Build history of the part. All positions in model axes, mm. Face numbers are marked on the shaded views. A direction names the side the tool comes from. Round coordinates to 2 decimals unless told otherwise and drop trailing zeros. Loops run counter-clockwise (first coordinate to the right, second up) from the corner with the lowest first, then second, coordinate; pieces in that order, holes last. Notation, with made-up numbers: M 87,12.25 L 121,12.25 A20 ccw 121,51.25 Z; hole C -24,40.5 d6. An arc over 180 degrees is marked long. Write each question's results on one line, items separated by ' | '. Start each with the question number.
```python
from build123d import *

# Parameters (mm, degrees)
SLEEVE_DEPTH       = 63.5
SLEEVE_DEPTH_BACK  = 5
SKETCH1_R          = 9.525
SKETCH2_W          = 19.05
SKETCH2_H          = 6.35
BRACKET_DEPTH      = 122
SKETCH4_R          = 5.1
BRACKET_HOLE_DEPTH = 138.86578845
SKETCH5_R          = 6.35
SHAFT_DEPTH        = 75
SKETCH6_R          = 8.73125
SLEEVE_HOLE_DEPTH  = 157.656471388
FILLET1_R          = 5


with BuildPart() as part:
    # Sketch1 → Sleeve (new, two sides: drawn at the far end of the back side and taken through both)
    with BuildSketch(Plane(origin=(0, 0, 0), x_dir=(1, 0, 0), z_dir=(0, 1, 0)).offset(-SLEEVE_DEPTH_BACK)):
        with Locations(Location((0, 0, 0), (0, 0, 270))):
            Circle(SKETCH1_R)
    extrude(amount=SLEEVE_DEPTH + SLEEVE_DEPTH_BACK)

    # Sketch2 → Bracket (add)
    with BuildSketch(Plane.XY):
        with Locations((0, 53.5)):
            Rectangle(SKETCH2_W, SKETCH2_H)
    extrude(amount=BRACKET_DEPTH)

    # Sketch4 → Bracket Hole (cut, through all)
    with BuildSketch(Plane(origin=(0, 0, 0), x_dir=(1, 0, 0), z_dir=(0, 1, 0))):
        with Locations(Location((0, -50.8, 0), (0, 0, 90))):
            Circle(SKETCH4_R)
        with Locations(Location((0, -66.1, 0), (0, 0, 90))):
            Circle(SKETCH4_R)
        with Locations(Location((0, -81.4, 0), (0, 0, 90))):
            Circle(SKETCH4_R)
        with Locations(Location((0, -96.7, 0), (0, 0, 90))):
            Circle(SKETCH4_R)
        with Locations(Location((0, -112, 0), (0, 0, 90))):
            Circle(SKETCH4_R)
    extrude(amount=BRACKET_HOLE_DEPTH, mode=Mode.SUBTRACT)

    # Sketch5 → Shaft (add)
    with BuildSketch(Plane(origin=(0, 0, 0), x_dir=(0, 0, -1), z_dir=(1, 0, 0))):
        with Locations(Location((0, 10, 0), (0, 0, 180))):
            Circle(SKETCH5_R)
    extrude(amount=SHAFT_DEPTH)

    # Sketch6 → Sleeve Hole (cut, through all)
    with BuildSketch(Plane(origin=(0, 0, 0), x_dir=(1, 0, 0), z_dir=(0, 1, 0))):
        with Locations(Location((0, 0, 0), (0, 0, 270))):
            Circle(SKETCH6_R)
    extrude(amount=SLEEVE_HOLE_DEPTH, mode=Mode.SUBTRACT)

    # Fillet1
    fillet1_edges = [part.edges().sort_by_distance(p)[0] for p in [
        (-9.525, 53.5, 122),
        (9.525, 53.5, 122),
    ]]
    fillet(fillet1_edges, radius=FILLET1_R)


solid = part.part
```
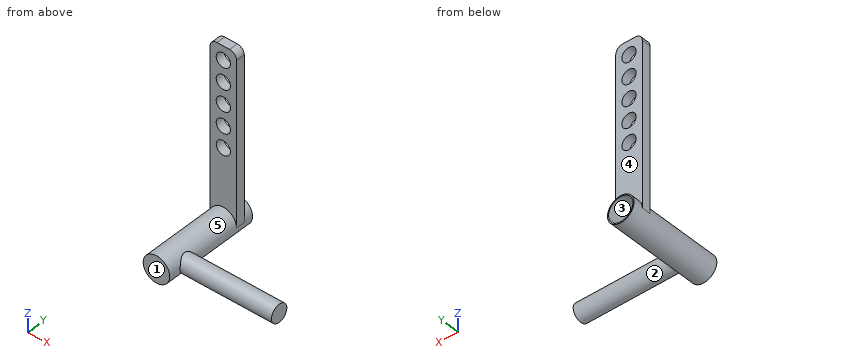
Item 1: Drop flat-ended pins along their axis: pin 1 (9 mm diameter, centred on x = 0, z = 66.1, fed in from -Y); pin 2 (1.9 mm diameter, centred on y = 53, z = 80.5, fed in from +X) (3 decimals); pin 3 (21 mm diameter, centred on x = -4, z = 89, fed in from +Y) (3 decimals); pin 4 (8.5 mm diameter, centred on x = -2.5, z = -2, fed in from +Y). Give the stop position or say it passes through.
Item 2: Drill centre lines: line 1 along X through (y, z) = (53.5, 81.4) (3 decimals); line 2 along Y through (x, z) = (3, 45) (3 decimals); line 3 along Z through (x, y) = (1, 37). Where is each one in solid material? Low to high. Write a range as [from, to].
Item 3: Saw through at A-A, the plane z = 112. Give the cut face in (x, y) (3 decimals).
Item 4: Saw through at D-D, the plane z = 66.5. Give the cut face in (x, y) (3 decimals).
Item 5: Mould opens along X. For the marked faces 3, 4 and 5 say: released by +X, released by -X, zero draft, split by the parting line, or undercut.
Item 6: Saw through at C-C, the plane x = 29.5. Give the cut face in (y, z), then the cut area to 3 significant figures.
Item 7: Tool access for the marked faces 1 and 2: list every direction of +Z, -Z, +X, -X, +Y, -Y with a clear straight run to the whole face (end or side of a thin tool).
Working result:
1) pin 1: passes through | pin 2: stops at x = 9.525 | pin 3: stops at y = 56.675 | pin 4: stops at y = 0
2) line 1: x = [-9.525, -5.1], [5.1, 9.525] | line 2: y = [50.325, 56.675] | line 3: z = [-9.47, -8.67], [8.67, 9.47]
3) outline: M -9.525,50.325 L -5.1,50.325 L -5.1,56.675 L -9.525,56.675 Z; M 5.1,50.325 L 9.525,50.325 L 9.525,56.675 L 5.1,56.675 Z
4) outline: M -9.525,50.325 L -5.084,50.325 L -5.084,56.675 L -9.525,56.675 Z; M 5.084,50.325 L 9.525,50.325 L 9.525,56.675 L 5.084,56.675 Z
5) face 3: undercut | face 4: zero draft | face 5: split by the parting line
6) outline: C 10,0 d12.7 | area: 127 mm²
7) face 1: +Z, -Z, +X, -X, -Y | face 2: +X
